```python
from build123d import *

# Parameters (mm, degrees)
SKETCH_1_W          = 27.5
SKETCH_1_H          = 45
SKETCH_1_R          = 1
EXTRUDE_1_DEPTH     = 15
SKETCH_2_R          = 2.526456565
CUT_EXTRUDE_1_DEPTH = 1


with BuildPart() as part:
    # 草图1 → 凸台-拉伸1 (new body)
    with BuildSketch(Plane(origin=(0, 0, 0), x_dir=(1, 0, 0), z_dir=(0, 1, 0))):
        Rectangle(SKETCH_1_W, SKETCH_1_H)
        with Locations(Location((-12.3, 15.1, 0), (0, 0, 270))):
            Circle(SKETCH_1_R, mode=Mode.SUBTRACT)
        with Locations(Location((12.3, 15.1, 0), (0, 0, 270))):
            Circle(SKETCH_1_R, mode=Mode.SUBTRACT)
        with Locations(Location((12.3, -11.3, 0), (0, 0, 270))):
            Circle(SKETCH_1_R, mode=Mode.SUBTRACT)
        with Locations(Location((-12.3, -11.3, 0), (0, 0, 270))):
            Circle(SKETCH_1_R, mode=Mode.SUBTRACT)
    extrude(amount=EXTRUDE_1_DEPTH)

    # 草图2 → 切除-拉伸1 (cut)
    with BuildSketch(Plane.XY.offset(22.5)):
        with Locations((0, 7.614868715)):
            Circle(SKETCH_2_R)
    extrude(amount=-CUT_EXTRUDE_1_DEPTH, mode=Mode.SUBTRACT)


solid = part.part
```
For this review, take the finished solid that the model builds, in its own axes (mm). A direction names the side the tool comes from. Round coordinates to 2 decimals unless told otherwise and drop trailing zeros. Write each loop counter-clockwise with the first axis right and the second up, starting at its lowest first coordinate (ties: lowest second). Pieces come first, ordered by that corner, then holes. Notation, with made-up numbers: (25.5, 56.25) - (80.5, 56.25) arc R19 cw to (80.5, 87.25) - close; hole circle Ø6 at (26, 52). An arc over 180 degrees is marked (long way). Write each question's results on one line, items separated by ' | '.
Item 1: Take a section at B-B on z = -15.1. State the section outline as (x, y) points, then the cut area to 4 significant figures.
Calculated:
outline: (-13.75, 0) - (-13.3, 0) - (-13.3, 15) - (-13.75, 15) - close; (-11.3, 0) - (11.3, 0) - (11.3, 15) - (-11.3, 15) - close; (13.3, 0) - (13.75, 0) - (13.75, 15) - (13.3, 15) - close | area: 352.5 mm^2
Item 2: For pin 1 (2.5 mm diameter, centred on x = -0.5, y = 7.5, fed in from +Z); pin 2 (1.2 mm diameter, centred on x = -12.3, z = 11.3, fed in from -Y); pin 3 (2.5 mm diameter, centred on x = 12.3, z = -15.1, fed in from +Y), all flat-tipped, find the tip position at first contact; note any pin that passes through.
Calculated:
pin 1: stops at z = 21.5 | pin 2: passes through | pin 3: stops at y = 15
Item 3: To check wall thickness, follow line 1 along X through (y, z) = (8.25, -15.1); line 2 along Y through (x, z) = (0, 21.8); line 3 along X through (y, z) = (8.75, -15.5). State the ranges of each line that lie inside material, in increasing order. Write a range as from..to.
Calculated:
line 1: x = -13.75..-13.3, -11.3..11.3, 13.3..13.75 | line 2: y = 0..5.09, 10.14..15 | line 3: x = -13.75..-13.22, -11.38..11.38, 13.22..13.75
Item 4: Draft analysis for pull direction X (two halves, no side actions). For faces 3 (the face through (1.358, 9.745, 22.007)), 4 (the face through (13.75, 7, 0)), 5 (the face through (11.917, 7.395, 12.224)), 6 (the face through (0, 15, 0)), state which applies: pulls with the +X half, pulls with the -X half, needs draft (parallel to the pull), parting line crosses it, or undercut.
Calculated:
face 3: undercut | face 4: pulls with the +X half | face 5: undercut | face 6: needs draft
Item 5: For faces 1 (the face through (0, 8, 21.5)), 2 (the face through (0, 0, 0)), list the 3-axis set-ups (+Z, -Z, +X, -X, +Y, -Y) from which the entire face can be reached by the end or side of a thin tool; tool diameter is ignored.
Calculated:
face 1: +Z | face 2: +Z, -Z, +X, -X, -Y
Item 6: Take a section at A-A on x = -12.3. State the section outline as (y, z) points.
Calculated:
outline: (0, -22.5) - (15, -22.5) - (15, -16.1) - (0, -16.1) - close; (0, -14.1) - (15, -14.1) - (15, 10.3) - (0, 10.3) - close; (0, 12.3) - (15, 12.3) - (15, 22.5) - (0, 22.5) - close
